```python
from build123d import *
from OCP.BRepFilletAPI import BRepFilletAPI_MakeChamfer

# Parameters (mm, degrees)
SKETCH1_W           = 42
SKETCH1_H           = 42
SKETCH1_R           = 12
SKETCH1_R_2         = 1.5
BOSS_EXTRUDE1_DEPTH = 6
CHAMFER1_SIZE       = 2
SKETCH2_W           = 24
SKETCH2_H           = 21
CUT_EXTRUDE1_DEPTH  = 31.298514815
CHAMFER2_SIZE       = 4.5
CHAMFER2_SIZE2      = 1.205771366
BOSS_EXTRUDE2_DEPTH = 6
CUT_EXTRUDE2_DEPTH  = 43.107006543


with BuildPart() as part:
    # Sketch1 → Boss-Extrude1 (new body)
    with BuildSketch(Plane(origin=(0, 0, 0), x_dir=(1, 0, 0), z_dir=(0, 1, 0))):
        Rectangle(SKETCH1_W, SKETCH1_H)
        with Locations(Location((0, 0, 0), (0, 0, 270))):
            Circle(SKETCH1_R, mode=Mode.SUBTRACT)
        with Locations(Location((-15.5, 15.5, 0), (0, 0, 270))):
            Circle(SKETCH1_R_2, mode=Mode.SUBTRACT)
        with Locations(Location((15.5, 15.5, 0), (0, 0, 270))):
            Circle(SKETCH1_R_2, mode=Mode.SUBTRACT)
        with Locations(Location((15.5, -15.5, 0), (0, 0, 270))):
            Circle(SKETCH1_R_2, mode=Mode.SUBTRACT)
        with Locations(Location((-15.5, -15.5, 0), (0, 0, 270))):
            Circle(SKETCH1_R_2, mode=Mode.SUBTRACT)
    extrude(amount=BOSS_EXTRUDE1_DEPTH)

    # Chamfer1
    chamfer1_edges = [part.edges().sort_by_distance(p)[0] for p in [
        (21, 3, 21),
        (-21, 3, 21),
        (-21, 3, -21),
        (21, 3, -21),
    ]]
    chamfer(chamfer1_edges, length=CHAMFER1_SIZE)

    # Sketch2 → Cut-Extrude1 (cut, through all)
    with BuildSketch(Plane(origin=(0, 6, 0), x_dir=(1, 0, 0), z_dir=(0, 1, 0))):
        with Locations((0, -10.5)):
            Rectangle(SKETCH2_W, SKETCH2_H)
    extrude(amount=-CUT_EXTRUDE1_DEPTH, mode=Mode.SUBTRACT)

    # Chamfer2: one chamfer whose edges measure the first distance from different faces: ONE call of the kernel's chamfer builder (chamfer() names one face for all edges)
    chamfer2_edges_1 = [part.edges().sort_by_distance(p)[0] for p in [
        (12, 3, 21),
    ]]
    chamfer2_side_1 = [part.faces().sort_by_distance(p)[0] for p in [
        (12, 3, 10.5),
    ]]
    chamfer2_edges_2 = [part.edges().sort_by_distance(p)[0] for p in [
        (-12, 3, 21),
    ]]
    chamfer2_side_2 = [part.faces().sort_by_distance(p)[0] for p in [
        (-12, 3, 10.5),
    ]]
    chamfer2 = BRepFilletAPI_MakeChamfer(part.part.solid().wrapped)
    for e in chamfer2_edges_1:
        chamfer2.Add(CHAMFER2_SIZE, CHAMFER2_SIZE2, e.wrapped, chamfer2_side_1[0].wrapped)  # the first distance lies on this face
    for e in chamfer2_edges_2:
        chamfer2.Add(CHAMFER2_SIZE, CHAMFER2_SIZE2, e.wrapped, chamfer2_side_2[0].wrapped)  # the first distance lies on this face
    add(Compound.cast(chamfer2.Shape()), mode=Mode.REPLACE)

    # Sketch3 → Boss-Extrude2 (add)
    with BuildSketch(Plane(origin=(0, 6, 0), x_dir=(1, 0, 0), z_dir=(0, 1, 0))):
        with BuildLine():
            Line((0, 21), (6, 21))
            ThreePointArc((6, 21), (9, 24), (12, 21))
            Line((12, 21), (18, 21))
            ThreePointArc((18, 21), (9, 30), (0, 21))
        make_face()
    extrude(amount=-BOSS_EXTRUDE2_DEPTH)

    # Sketch4 → Cut-Extrude2 (cut, through all)
    with BuildSketch(Plane(origin=(0, 6, 6), x_dir=(1, 0, 0), z_dir=(0, 1, 0))):
        with BuildLine():
            Line((12, 6), (12, 27))
            ThreePointArc((12, 27), (9, 30), (6, 27))
            Line((6, 27), (6, 18))
            Line((6, 18), (0, 18))
            Line((0, 18), (0, 6))
            Line((0, 6), (12, 6))
        make_face()
    extrude(amount=-CUT_EXTRUDE2_DEPTH, mode=Mode.SUBTRACT)


solid = part.part
```
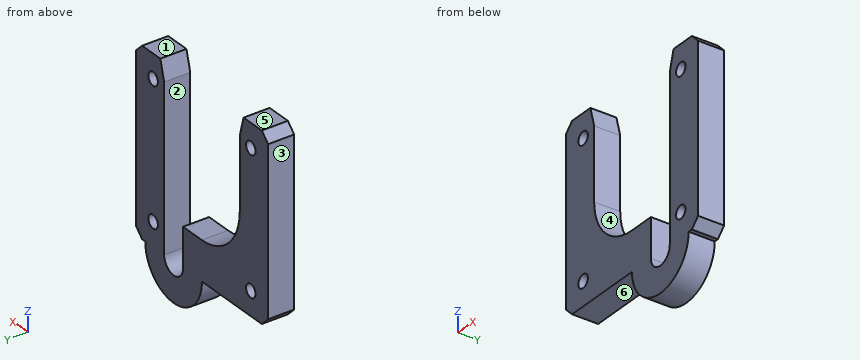
Model file for the job. Use its own axes, mm. Face numbers are marked on the shaded views. A direction names the side the tool comes from. Coordinates: 2 decimals unless noted, no trailing zeros. Order: outer loops, then holes, each group sorted by start corner. A loop starts at its lowest first (then second) coordinate and runs counter-clockwise, first axis right, second up. Notation, with made-up numbers: (-6, 34) -> (25, 34) arc R22 ccw to (25, 58) -> close; hole circle Ø4 at (18.25, -27). An arc over 180 degrees is marked (long way). Answer as a JSON object with one key per item and string values. Group by question number.
1) Cut at A-A, the plane z = 15.5. Write the cut outline in (x, y), then the cut area to 3 significant figures.
2) Cut at D-D, the plane z = -18. Write the cut outline in (x, y).
3) Pull direction X, two halves, no side cores. Call the marked faces 1, 2 and 3: +X half, -X half, draft (parallel to the pull), parting line (faces both ways), or undercut.
4) Cut at B-B, the plane y = 5.2. Write the cut outline in (x, z).
5) Which spindle directions (+Z, -Z, +X, -X, +Y, -Y) get a long thin tool onto all of the face, cutting with end or side? Do the marked faces 4, 5 and 6. Say none if no direction does.
6) Cut at C-C, the plane x = -15.5. Write the cut outline in (y, z).
7) Drill centre lines: L1, parallel to X at y = 3.25, z = 15.5; L2, parallel to X at y = 1.7, z = -15.5; L3, parallel to X at y = 0.6, z = 13. Where is each one in solid material? Low to high.
Check values:
{
 "1": {"outline": "(-21, 0) -> (-17, 0) -> (-17, 6) -> (-21, 6) -> close; (-14, 0) -> (-12, 0) -> (-12, 6) -> (-14, 6) -> close; (12, 0) -> (14, 0) -> (14, 6) -> (12, 6) -> close; (17, 0) -> (21, 0) -> (21, 6) -> (17, 6) -> close", "area": "72.0 mm²"},
 "2": {"outline": "(-21, 0) -> (6, 0) -> (6, 6) -> (-21, 6) -> close; (12, 0) -> (21, 0) -> (21, 6) -> (12, 6) -> close"},
 "3": {"face 1": "draft", "face 2": "undercut", "face 3": "-X half"},
 "4": {"outline": "(-21, -19) -> (-19, -21) -> (0, -21) arc R9 ccw to (18, -21) -> (19, -21) -> (21, -19) -> (21, 19) -> (19, 21) -> (13.21, 21) -> (12, 16.5) -> (12, -21) arc R3 cw to (6, -21) -> (6, -12) -> (0, -12) arc R12 cw to (-12, 0) -> (-12, 16.5) -> (-13.21, 21) -> (-19, 21) -> (-21, 19) -> close; hole circle Ø3 at (-15.5, -15.5); hole circle Ø3 at (-15.5, 15.5); hole circle Ø3 at (15.5, -15.5); hole circle Ø3 at (15.5, 15.5)"},
 "5": {"face 4": "+Z, +Y, -Y", "face 5": "+Z, +X, -X, +Y, -Y", "face 6": "-Z, -X, +Y, -Y"},
 "6": {"outline": "(0, -21) -> (6, -21) -> (6, -17) -> (0, -17) -> close; (0, -14) -> (6, -14) -> (6, 14) -> (0, 14) -> close; (0, 17) -> (6, 17) -> (6, 21) -> (0, 21) -> close"},
 "7": {"L1": "x = -21 to -17, -14 to -12, 12 to 14, 17 to 21", "L2": "x = -21 to -17, -14 to 6, 12 to 14, 17 to 21", "L3": "x = -21 to -12, 12 to 21"}
}
